Answer from the drawing. Dimensions are ordinates in mm from the lowest x, y and z of the part. A direction names the side the tool comes from. Coordinates: 2 decimals unless noted, no trailing zeros. Write each loop counter-clockwise with the first axis right and the second up, starting at its lowest first coordinate (ties: lowest second). Pieces come first, ordered by that corner, then holes. Notation, with made-up numbers: (8, 80) - (41, 80) arc R28 ccw to (41, 104) - close; hole circle Ø8 at (11.5, 42.5). An arc over 180 degrees is marked (long way). Return JSON: item names as keys, results as strings.
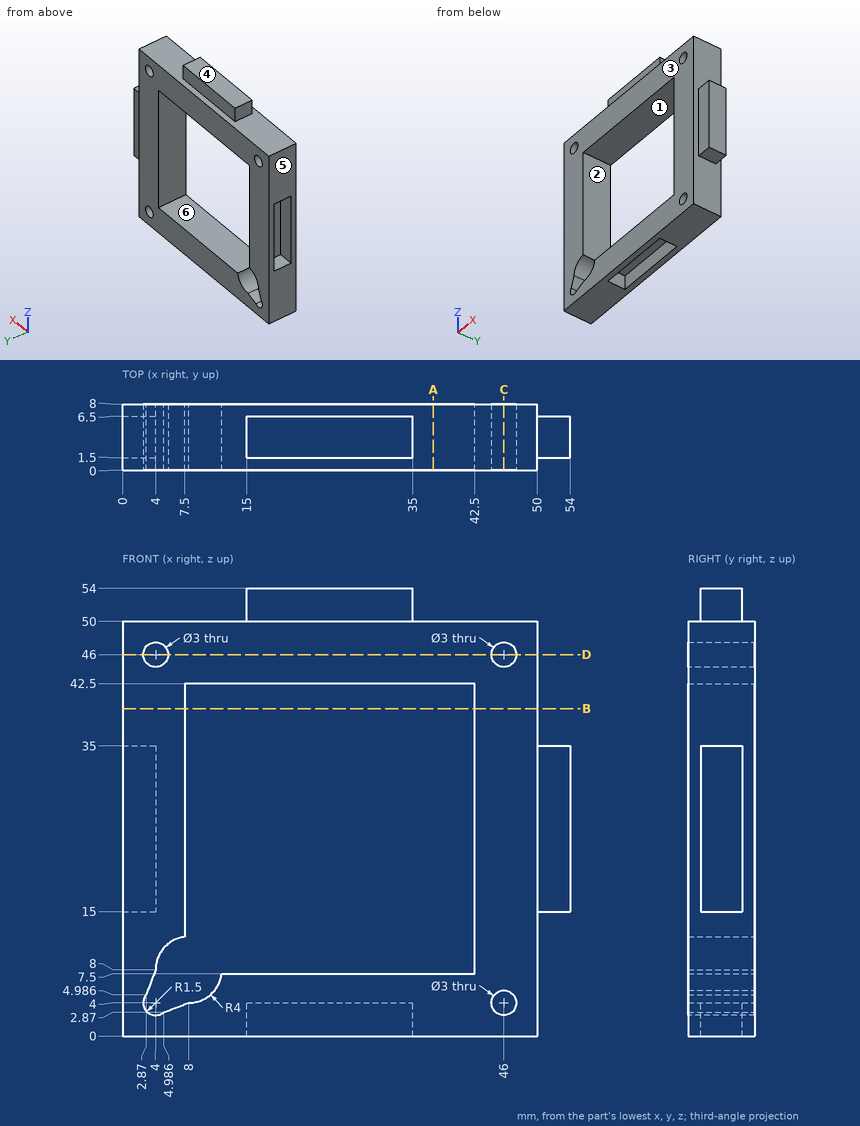
(1) A cutting plane is placed at A-A (x = 37.5). Determine the outline of the cut face in (y, z).
Answer:
{"outline": "(0, 0) - (8, 0) - (8, 7.5) - (0, 7.5) - close; (0, 42.5) - (8, 42.5) - (8, 50) - (0, 50) - close"}
(2) A cutting plane is placed at C-C (x = 46). Determine the outline of the cut face in (y, z).
Answer:
{"outline": "(0, 0) - (8, 0) - (8, 2.5) - (0, 2.5) - close; (0, 5.5) - (8, 5.5) - (8, 44.5) - (0, 44.5) - close; (0, 47.5) - (8, 47.5) - (8, 50) - (0, 50) - close"}
(3) Flat-ended cylindrical pins translate along their axes: P1, Ø3, axis at y = 4.5, z = 52.5, coming from the -X side; P2, Ø4.5, axis at y = 5, z = 53, coming from the +X side; P3, Ø1.2, axis at x = 52.5, z = 22, coming from the +Y side. Find the tip coordinate at first contact, or state that the pin passes through.
Answer:
{"P1": "x = 15", "P2": "x = 35", "P3": "y = 6.5"}
(4) A cutting plane is placed at B-B (z = 39.5). Determine the outline of the cut face in (x, y).
Answer:
{"outline": "(0, 0) - (7.5, 0) - (7.5, 8) - (0, 8) - close; (42.5, 0) - (50, 0) - (50, 8) - (42.5, 8) - close"}
(5) Determine the mould class of the marked faces 1, 2, 3 and 4 for opening direction Z: +Z half, -Z half, draft (parallel to the pull), parting line (faces both ways), or undercut.
Answer:
{"face 1": "undercut", "face 2": "undercut", "face 3": "draft", "face 4": "+Z half"}
(6) Which of the six approach directions +Z, -Z, +X, -X, +Y, -Y give full straight-line access (tool end or side, diameter ignored) to the marked faces 5 and 6?
Answer:
{"face 5": "+Z, -Z, -X, +Y, -Y", "face 6": "+Y, -Y"}
(7) A cutting plane is placed at D-D (z = 46). Determine the outline of the cut face in (x, y).
Answer:
{"outline": "(0, 0) - (2.5, 0) - (2.5, 8) - (0, 8) - close; (5.5, 0) - (44.5, 0) - (44.5, 8) - (5.5, 8) - close; (47.5, 0) - (50, 0) - (50, 8) - (47.5, 8) - close"}
(8) Straight lines are drawn through the part: line 1 (X direction, y = 4.5, z = 46); line 2 (X direction, y = 4.5, z = 29); line 3 (Z direction, x = 23, y = 1.25). For each, find the intervals that lie inside material, in ascending order. Write a range as from..to.
Answer:
{"line 1": "0..2.5, 5.5..44.5, 47.5..50", "line 2": "4..7.5, 42.5..54", "line 3": "0..7.5, 42.5..50"}
